Could you check a few things on this drawing? It's one solid part, dimensions in mm from its lowest x, y, z. Give positions to 0.01 mm unless a question says otherwise; leave off trailing zeros. Loops run counter-clockwise (first coordinate to the right, second up) from the corner with the lowest first, then second, coordinate; pieces in that order, holes last. Notation, with made-up numbers: M 79.25,-6 L 121.25,-6 A15 cw 121.25,17 Z; hole C 77,60 d10. An arc over 180 degrees is marked long. Answer as a JSON object with one key per item and string values.
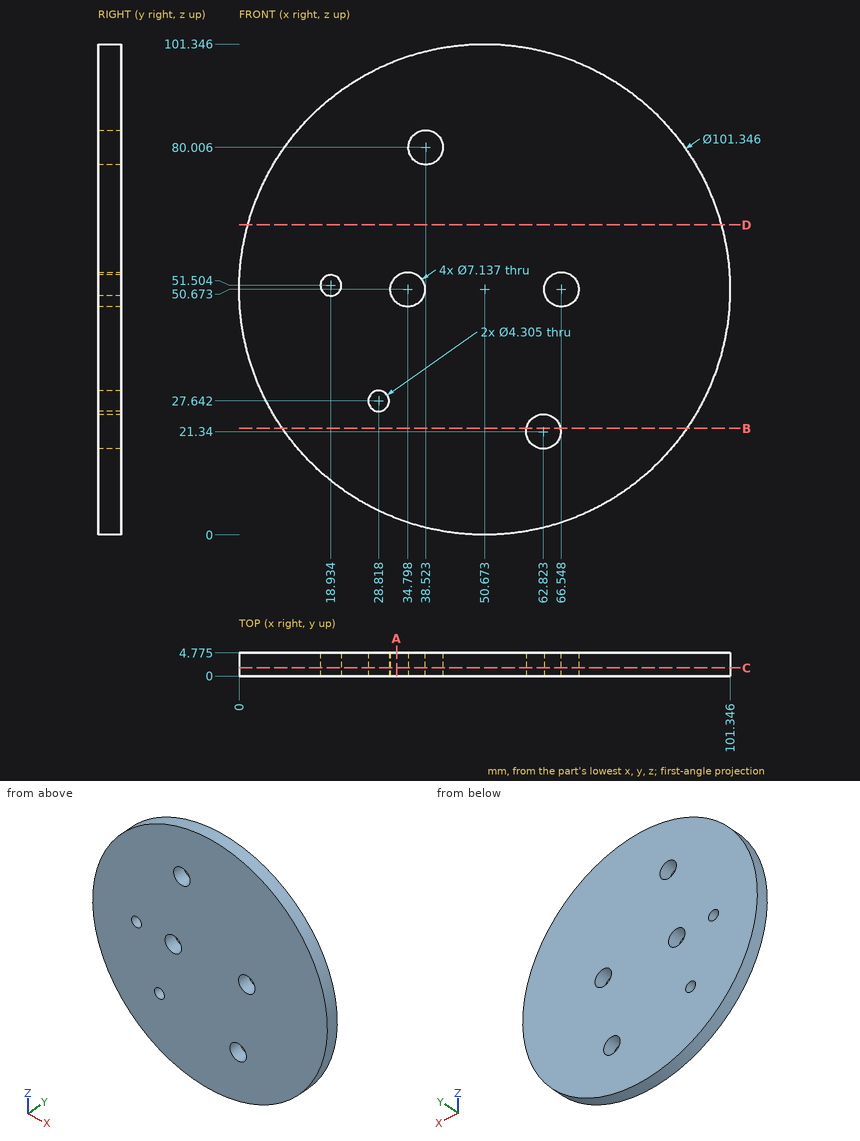
1) Suppose I cut it at D-D, the plane z = 64. Write out the boundary of the cut face in (x, y) (1 decimal).
Answer list:
{"outline": "M 1.8,0 L 99.6,0 L 99.6,4.8 L 1.8,4.8 Z"}
2) Suppose I cut it at C-C, the plane y = 1.7. Write out the boundary of the cut face in (x, z) (1 decimal), and give its area (3 significant figures).
Answer list:
{"outline": "C 50.7,50.7 d101.3; hole C 18.9,51.5 d4.3; hole C 28.8,27.6 d4.3; hole C 34.8,50.7 d7.1; hole C 38.5,80 d7.1; hole C 62.8,21.3 d7.1; hole C 66.5,50.7 d7.1", "area": "7,880 mm^2"}
3) Please list where these lines run through material, in increasing order: line 1 along Z through (x, y) = (37, 2.35) (1 decimal); line 2 along Z through (x, y) = (60, 2.85) (1 decimal); line 3 along X through (y, z) = (3.3, 77) (1 decimal). Write a range as from..to.
Answer list:
{"line 1": "1.9..47.9, 53.5..76.8, 83.2..99.5", "line 2": "0.9..19.2, 23.5..100.5", "line 3": "7.4..36.6, 40.4..94"}
4) Will these pins go through, and if not, where does the flat tip stop? pin 1 Ø5.5 at (x, z) = (18.93, 51.5) entering from -Y; pin 2 Ø6.5 at (x, z) = (66.548, 50.673) entering from -Y; pin 3 Ø1 at (x, y) = (27, 1) entering from -Z; pin 4 Ø1.5 at (y, z) = (4, 34.5) entering from +X.
Answer list:
{"pin 1": "y = 0", "pin 2": "through", "pin 3": "z = 5.61", "pin 4": "x = 98.94"}
5) Suppose I cut it at A-A, the plane x = 32.5. Write out the boundary of the cut face in (y, z) (1 decimal).
Answer list:
{"outline": "M 0,3.4 L 4.8,3.4 L 4.8,47.9 L 0,47.9 Z; M 0,53.4 L 4.8,53.4 L 4.8,98 L 0,98 Z"}
6) Suppose I cut it at B-B, the plane z = 22. Write out the boundary of the cut face in (x, y) (1 decimal).
Answer list:
{"outline": "M 8.9,0 L 59.3,0 L 59.3,4.8 L 8.9,4.8 Z; M 66.3,0 L 92.5,0 L 92.5,4.8 L 66.3,4.8 Z"}
